Model file for the job. Use its own axes, mm. A direction names the side the tool comes from. Give positions to 0.01 mm unless a question says otherwise; leave off trailing zeros. Write each loop counter-clockwise with the first axis right and the second up, starting at its lowest first coordinate (ties: lowest second). Pieces come first, ordered by that corner, then holes.
```python
from build123d import *

# Parameters (mm, degrees)
SKETCH1_W           = 47
SKETCH1_H           = 32
SKETCH1_W_2         = 43
SKETCH1_H_2         = 28
BOSS_EXTRUDE1_DEPTH = 28
SKETCH2_W           = 44
SKETCH2_H           = 29
CUT_EXTRUDE1_DEPTH  = 10
SKETCH3_W           = 47
SKETCH3_H           = 32
SKETCH3_W_2         = 44
SKETCH3_H_2         = 29
BOSS_EXTRUDE2_DEPTH = 25
SKETCH4_W           = 47
SKETCH4_H           = 32
SKETCH4_R           = 6.5
BOSS_EXTRUDE3_DEPTH = 3
SKETCH5_R           = 5
SKETCH5_R_2         = 4
BOSS_EXTRUDE4_DEPTH = 5
SKETCH6_R           = 2.65
BOSS_EXTRUDE5_DEPTH = 5


with BuildPart() as part:
    # Sketch1 → Boss-Extrude1 (new body)
    with BuildSketch(Plane(origin=(0, 0, 0), x_dir=(1, 0, 0), z_dir=(0, 1, 0))):
        with Locations((23.5, 16)):
            Rectangle(SKETCH1_W, SKETCH1_H)
        with Locations((23.5, 16)):
            Rectangle(SKETCH1_W_2, SKETCH1_H_2, mode=Mode.SUBTRACT)
    extrude(amount=BOSS_EXTRUDE1_DEPTH)

    # Sketch2 → Cut-Extrude1 (cut)
    with BuildSketch(Plane.XZ):
        with Locations((23.5, -16)):
            Rectangle(SKETCH2_W, SKETCH2_H)
    extrude(amount=-CUT_EXTRUDE1_DEPTH, mode=Mode.SUBTRACT)

    # Sketch3 → Boss-Extrude2 (add)
    with BuildSketch(Plane.XZ):
        with Locations((23.5, -16)):
            Rectangle(SKETCH3_W, SKETCH3_H)
        with Locations((23.5, -16)):
            Rectangle(SKETCH3_W_2, SKETCH3_H_2, mode=Mode.SUBTRACT)
    extrude(amount=BOSS_EXTRUDE2_DEPTH)

    # Sketch4 → Boss-Extrude3 (add)
    with BuildSketch(Plane.XZ.offset(25)):
        with Locations((23.5, -16)):
            Rectangle(SKETCH4_W, SKETCH4_H)
        with Locations(Location((23.5, -16, 0), (0, 0, 270))):
            Circle(SKETCH4_R, mode=Mode.SUBTRACT)
    extrude(amount=-BOSS_EXTRUDE3_DEPTH)

    # Sketch5 → Boss-Extrude4 (add)
    # profile 1 of 2: a face of its own
    with BuildSketch(Plane.XZ.offset(25)):
        with Locations(Location((10, -16, 0), (0, 0, 270))):
            Circle(SKETCH5_R)
        with Locations(Location((10, -16, 0), (0, 0, 270))):
            Circle(SKETCH5_R_2, mode=Mode.SUBTRACT)
    # profile 2 of 2: a face of its own
    with BuildSketch(Plane.XZ.offset(25)):
        with Locations(Location((37, -16, 0), (0, 0, 270))):
            Circle(SKETCH5_R)
        with Locations(Location((37, -16, 0), (0, 0, 270))):
            Circle(SKETCH5_R_2, mode=Mode.SUBTRACT)
    extrude(amount=-BOSS_EXTRUDE4_DEPTH)

    # Sketch6 → Boss-Extrude5 (add)
    with BuildSketch(Plane.XZ.offset(25)):
        with Locations(Location((10, -16, 0), (0, 0, 270))):
            Circle(SKETCH6_R)
        with Locations(Location((37, -16, 0), (0, 0, 270))):
            Circle(SKETCH6_R)
    extrude(amount=-BOSS_EXTRUDE5_DEPTH)


solid = part.part
```
1. Pin check, flat tips, straight feed: P1, Ø7, axis at x = 37, z = -16, coming from the +Y side; P2, Ø2, axis at x = 29.5, z = -22, coming from the +Y side. Stop position of each tip, or through.
Calculated:
P1: stops at y = -20
P2: stops at y = -22
2. Pull direction X, two halves, no side cores. Call faces 4 (the flat face through (0, 2, -16)), 5 (the flat face through (23, 2, 0)), 6 (the cylindrical face through (10, -21, -12)): +X half, -X half, draft (parallel to the pull), parting line (faces both ways), or undercut.
Calculated:
face 4: -X half
face 5: draft
face 6: undercut
3. Slice it at B-B, the plane x = 23.5. Write the cut outline in (y, z), and give its area (3 significant figures).
Calculated:
outline: (-25, -32) - (28, -32) - (28, -30) - (10, -30) - (10, -30.5) - (-22, -30.5) - (-22, -22.5) - (-25, -22.5) - close; (-25, -9.5) - (-22, -9.5) - (-22, -1.5) - (10, -1.5) - (10, -2) - (28, -2) - (28, 0) - (-25, 0) - close
area: 225 mm2
4. Slice it at D-D, the plane x = 10. Write the cut outline in (y, z), and give its area (3 significant figures).
Calculated:
outline: (-25, -32) - (28, -32) - (28, -30) - (10, -30) - (10, -30.5) - (-22, -30.5) - (-22, -21) - (-20, -21) - (-20, -20) - (-22, -20) - (-22, -18.65) - (-20, -18.65) - (-20, -13.35) - (-22, -13.35) - (-22, -12) - (-20, -12) - (-20, -11) - (-22, -11) - (-22, -1.5) - (10, -1.5) - (10, -2) - (28, -2) - (28, 0) - (-25, 0) - close
area: 279 mm2
5. Slice it at C-C, the plane z = -29. Write the cut outline in (x, y).
Calculated:
outline: (0, -25) - (47, -25) - (47, 28) - (45, 28) - (45, 10) - (45.5, 10) - (45.5, -22) - (1.5, -22) - (1.5, 10) - (2, 10) - (2, 28) - (0, 28) - close
6. Slice it at A-A, the plane y = -16. Write the cut outline in (x, z), and give its area (3 significant figures).
Calculated:
outline: (0, -32) - (47, -32) - (47, 0) - (0, 0) - close; hole (1.5, -30.5) - (45.5, -30.5) - (45.5, -1.5) - (1.5, -1.5) - close
area: 228 mm2
7. Probe probe 1 along X at (y, z) = (-5.5, -29.5); probe 2 along X at (y, z) = (24.5, -15); probe 3 along Z at (x, y) = (8.5, -5). List the from-to ranges inside material, lowest first.
Calculated:
probe 1: x = 0 to 1.5, 45.5 to 47
probe 2: x = 0 to 2, 45 to 47
probe 3: z = -32 to -30.5, -1.5 to 0
8. Which spindle directions (+Z, -Z, +X, -X, +Y, -Y) get a long thin tool onto all of the face, cutting with end or side? Do faces 1 (the flat face through (23, -6, -30.5)), 2 (the cylindrical face through (39.234, -21.014, -17.425)), 3 (the flat face through (23, 28, -1)). Say none if no direction does.
Calculated:
face 1: none
face 2: +Y
face 3: +Z, -Z, +X, -X, +Y
